Design review of the part shown in the three views and the two pictorial views. Dimensions are in mm from the part's minimum x, y and z. Coordinates: 2 decimals unless noted, no trailing zeros. Write each loop counter-clockwise with the first axis right and the second up, starting at its lowest first coordinate (ties: lowest second). Pieces come first, ordered by that corner, then holes.
Q1. For L1, parallel to Y at x = 2.5, z = 359; L2, parallel to Y at x = 4.5, z = 124.5; L3, parallel to Z at x = 23, y = 49.5, list the stretches that pass through material, from the lowest coordinate up.
Q2. Take a section at B-B, the plane z = 345.5. Write out the cut boundary in (x, y).
Q3. For pin 1 Ø8 at (x, z) = (23, 141) entering from +Y, flat-tipped, find the tip position at first contact; note if it passes through.
Q4. Take a section at A-A, the plane z = 89.5. Write out the cut boundary in (x, y), plus the area to 4 significant figures.
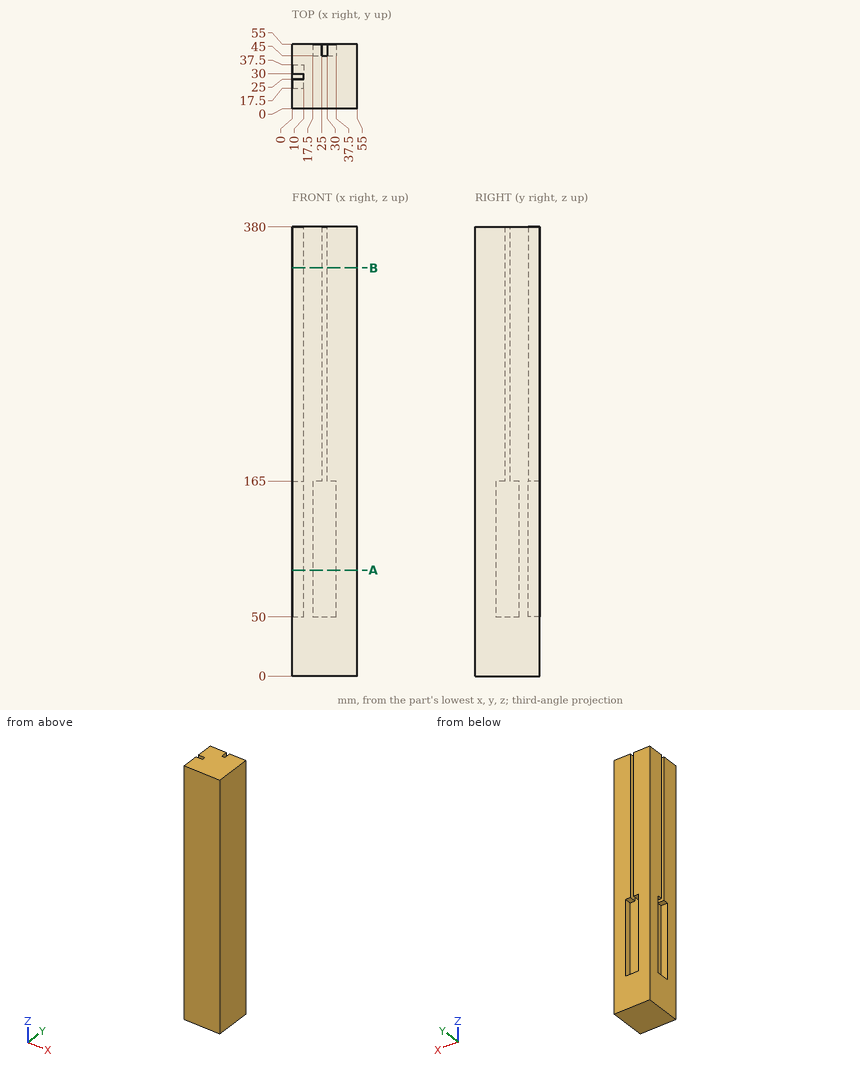
Responses:
1. L1: y = 0 to 25, 30 to 55
1. L2: y = 0 to 17.5, 37.5 to 55
1. L3: z = 0 to 50, 165 to 380
2. outline: (0, 0) - (55, 0) - (55, 55) - (30, 55) - (30, 45) - (25, 45) - (25, 55) - (0, 55) - (0, 30) - (10, 30) - (10, 25) - (0, 25) - close
3. pin 1: stops at y = 45
4. outline: (0, 0) - (55, 0) - (55, 55) - (37.5, 55) - (37.5, 45) - (17.5, 45) - (17.5, 55) - (0, 55) - (0, 37.5) - (10, 37.5) - (10, 17.5) - (0, 17.5) - close
4. area: 2,625 mm2
